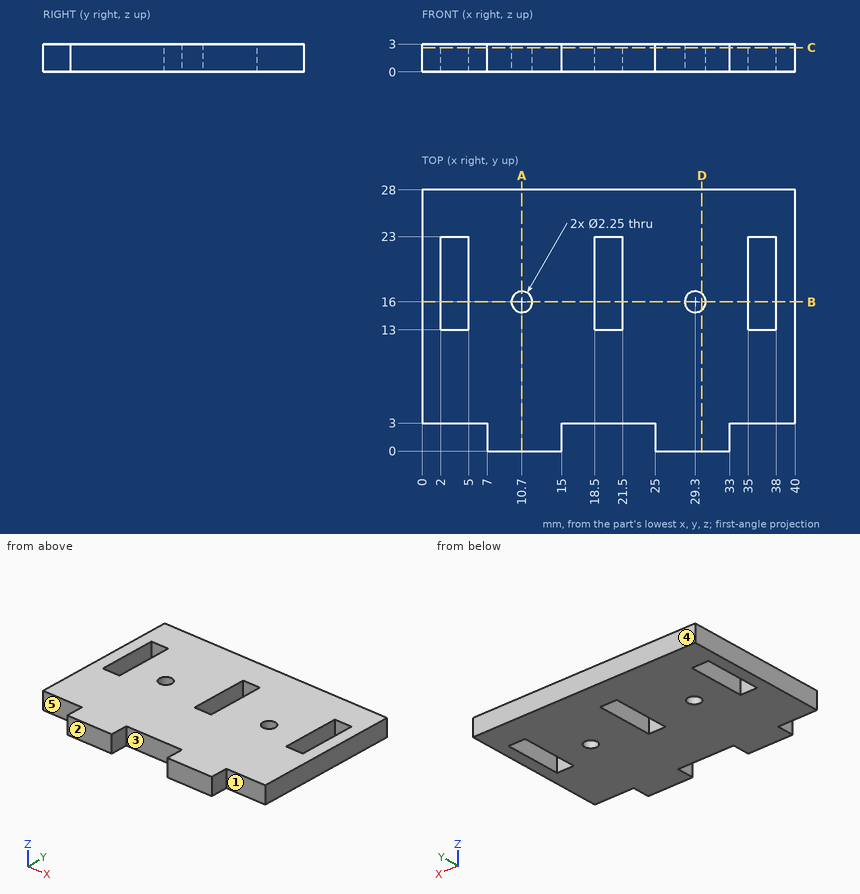
Part print with two shaded views. Sizes in mm from the minimum x, y, z corner. A direction names the side the tool comes from. Round coordinates to 2 decimals unless told otherwise and drop trailing zeros. Order: outer loops, then holes, each group sorted by start corner. A loop starts at its lowest first (then second) coordinate and runs counter-clockwise, first axis right, second up. Notation, with made-up numbers: (58, 57) - (104, 57) arc R21 ccw to (104, 74) - close; hole circle Ø2 at (-3.5, -38). An arc over 180 degrees is marked (long way). Return JSON: item names as keys, results as strings.
(1) Cut at D-D (x = 30). Give the cut face in (y, z), then the cut area to 3 significant figures.
Answer key:
{"outline": "(0, 0) - (15.12, 0) - (15.12, 3) - (0, 3) - close; (16.88, 0) - (28, 0) - (28, 3) - (16.88, 3) - close", "area": "78.7 mm^2"}
(2) Cut at C-C (z = 2.6). Give the cut face in (x, y) (3 decimals), then the cut area to 3 significant figures.
Answer key:
{"outline": "(0, 3) - (7, 3) - (7, 0) - (15, 0) - (15, 3) - (25, 3) - (25, 0) - (33, 0) - (33, 3) - (40, 3) - (40, 28) - (0, 28) - close; hole (2, 13) - (5, 13) - (5, 23) - (2, 23) - close; hole circle Ø2.25 at (10.7, 16); hole (18.5, 13) - (21.5, 13) - (21.5, 23) - (18.5, 23) - close; hole circle Ø2.25 at (29.3, 16); hole (35, 13) - (38, 13) - (38, 23) - (35, 23) - close", "area": "950 mm^2"}
(3) Tool access for the marked faces 1, 2, 3, 4 and 5: list every direction of +Z, -Z, +X, -X, +Y, -Y with a clear straight run to the whole face (end or side of a thin tool).
Answer key:
{"face 1": "+Z, -Z, +X, -Y", "face 2": "+Z, -Z, +X, -X, -Y", "face 3": "+Z, -Z, -Y", "face 4": "+Z, -Z, +X, -X, +Y", "face 5": "+Z, -Z, -X, -Y"}
(4) Cut at A-A (x = 10.7). Give the cut face in (y, z) (3 decimals), then the cut area to 4 significant figures.
Answer key:
{"outline": "(0, 0) - (14.875, 0) - (14.875, 3) - (0, 3) - close; (17.125, 0) - (28, 0) - (28, 3) - (17.125, 3) - close", "area": "77.25 mm^2"}
(5) Pin check, flat tips, straight feed: pin 1 Ø1.5 at (x, z) = (36.5, 1.5) entering from -Y; pin 2 Ø0.9 at (y, z) = (2, 2) entering from -X. Stop position of each tip, or through.
Answer key:
{"pin 1": "stops at y = 3", "pin 2": "stops at x = 7"}
(6) Wall check: probe 1 along X at (y, z) = (20.5, 2.2); probe 2 along Y at (x, z) = (29.3, 1.6) (3 decimals); probe 3 along Y at (x, z) = (21, 0.7). Give the ranges that are in metal, low to high. Write a range as from..to.
Answer key:
{"probe 1": "x = 0..2, 5..18.5, 21.5..35, 38..40", "probe 2": "y = 0..14.875, 17.125..28", "probe 3": "y = 3..13, 23..28"}
(7) Cut at B-B (y = 16). Give the cut face in (x, z) (3 decimals).
Answer key:
{"outline": "(0, 0) - (2, 0) - (2, 3) - (0, 3) - close; (5, 0) - (9.575, 0) - (9.575, 3) - (5, 3) - close; (11.825, 0) - (18.5, 0) - (18.5, 3) - (11.825, 3) - close; (21.5, 0) - (28.175, 0) - (28.175, 3) - (21.5, 3) - close; (30.425, 0) - (35, 0) - (35, 3) - (30.425, 3) - close; (38, 0) - (40, 0) - (40, 3) - (38, 3) - close"}
